from build123d import *

# Parameters (mm, degrees)
BOSS_EXTRUDE1_DEPTH      = 101.6
SKETCH2_R                = 6.35
BOSS_EXTRUDE2_DEPTH      = 127
BOSS_EXTRUDE2_DEPTH_BACK = 127


with BuildPart() as part:
    # Sketch1 → Boss-Extrude1 (new body, symmetric)
    with BuildSketch(Plane.XY):
        Polygon((0, 10.998522628), (-9.525, 5.499261314), (-9.525, -5.499261314), (0, -10.998522628), (9.525, -5.499261314), (9.525, 5.499261314), align=None)
    extrude(amount=BOSS_EXTRUDE1_DEPTH, both=True)

    # Sketch2 → Boss-Extrude2 (add, two sides)
    with BuildSketch(Plane.XY) as boss_extrude2_sk:
        Circle(SKETCH2_R)
    extrude(amount=BOSS_EXTRUDE2_DEPTH)
    extrude(boss_extrude2_sk.sketch, amount=-BOSS_EXTRUDE2_DEPTH_BACK)


solid = part.part
Model file for the job. Use its own axes, mm. A direction names the side the tool comes from. Round coordinates to 2 decimals unless told otherwise and drop trailing zeros. Loops run counter-clockwise (first coordinate to the right, second up) from the corner with the lowest first, then second, coordinate; pieces in that order, holes last. Notation, with made-up numbers: (-7, -23.5) - (28, -23.5) arc R33 cw to (28, 7.5) - close; hole circle Ø11 at (46.5, 73). An arc over 180 degrees is marked (long way). Write each question's results on one line, items separated by ' | '.
(1) Pin check, flat tips, straight feed: pin 1 (2 mm diameter, centred on x = -7.5, z = -17.5, fed in from +Y); pin 2 (1.5 mm diameter, centred on x = -2.5, z = -94.5, fed in from -Y); pin 3 (2 mm diameter, centred on x = -4, y = 6.5, fed in from -Z). Stop position of each tip, or through.
Answer below:
pin 1: stops at y = 7.25 | pin 2: stops at y = -9.99 | pin 3: stops at z = -101.6
(2) Saw through at A-A, the plane y = 0. List the corners of the cut face in (x, z) (3 decimals).
Answer below:
outline: (-9.525, -101.6) - (-6.35, -101.6) - (-6.35, -127) - (6.35, -127) - (6.35, -101.6) - (9.525, -101.6) - (9.525, 101.6) - (6.35, 101.6) - (6.35, 127) - (-6.35, 127) - (-6.35, 101.6) - (-9.525, 101.6) - close
(3) Saw through at B-B, the plane z = 80.5. List the corners of the cut face in (x, y) (3 decimals), then the cut area to 3 significant figures.
Answer below:
outline: (-9.525, -5.499) - (0, -10.999) - (9.525, -5.499) - (9.525, 5.499) - (0, 10.999) - (-9.525, 5.499) - close | area: 314 mm^2
(4) Wall check: L1, parallel to Z at x = -3.5, y = 7.25; L2, parallel to X at y = 7, z = -51; L3, parallel to X at y = 9.75, z = -12.5. Give the ranges that are in metal, low to high.
Answer below:
L1: z = -101.6 to 101.6 | L2: x = -6.93 to 6.93 | L3: x = -2.16 to 2.16
(5) 3-axis set-ups, long thin cutter, end or side, ignore diameter. For faces 1 (the cylindrical face through (-1.38, -6.2, -114.12)), 2 (the cylindrical face through (-1.38, -6.2, 114.12)), 3 (the flat face through (0, 0, -127)): which of +Z, -Z, +X, -X, +Y, -Y reach the whole face in a straight line?
Answer below:
face 1: -Z | face 2: +Z | face 3: -Z, +X, -X, +Y, -Y
(6) Saw through at C-C, the plane x = 2.5. List the corners of the cut face in (y, z).
Answer below:
outline: (-9.56, -101.6) - (-5.84, -101.6) - (-5.84, -127) - (5.84, -127) - (5.84, -101.6) - (9.56, -101.6) - (9.56, 101.6) - (5.84, 101.6) - (5.84, 127) - (-5.84, 127) - (-5.84, 101.6) - (-9.56, 101.6) - close
